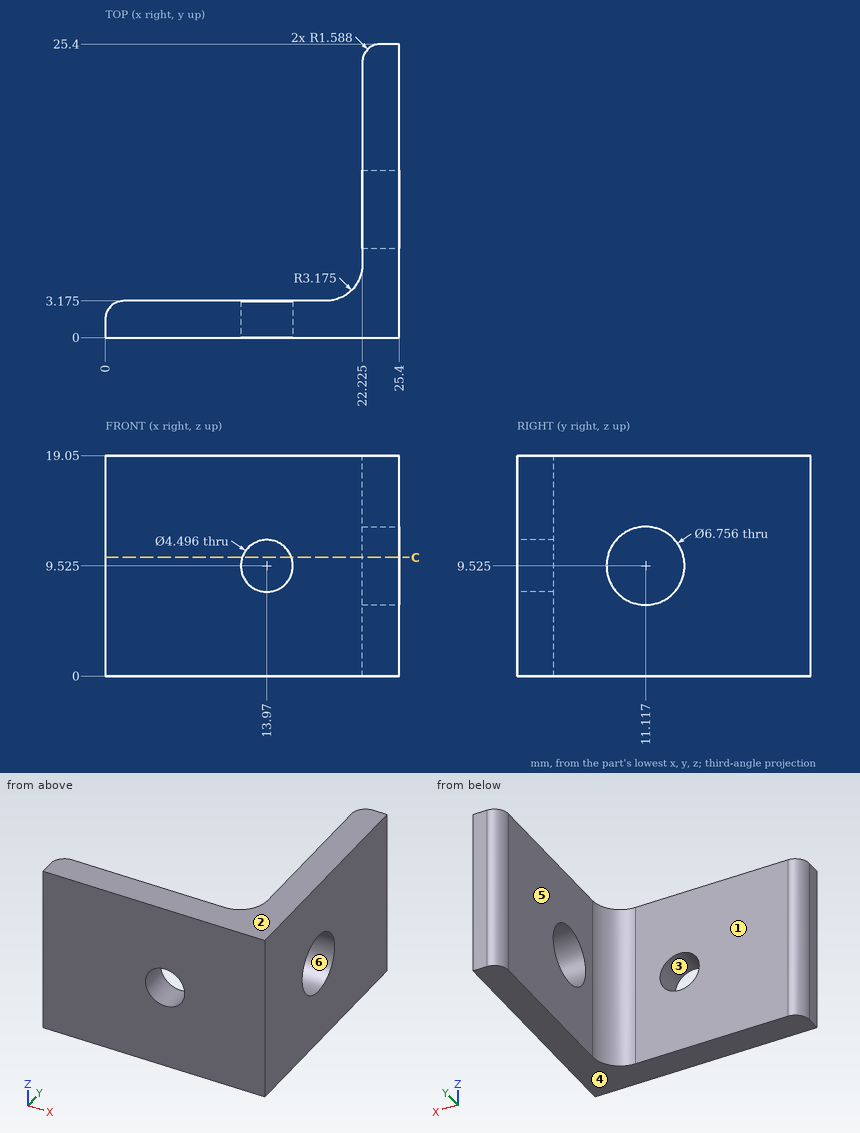
Part print with two shaded views. Sizes in mm from the minimum x, y, z corner. A direction names the side the tool comes from. Round coordinates to 2 decimals unless told otherwise and drop trailing zeros. Write each question's results on one line, items separated by ' | '.
1. Pull direction Z, two halves, no side cores. Call the marked faces 1, 2, 3 and 4: pulls with the +Z half, pulls with the -Z half, needs draft (parallel to the pull), parting line crosses it, or undercut.
Findings below:
face 1: needs draft | face 2: pulls with the +Z half | face 3: undercut | face 4: pulls with the -Z half
2. Wall check: line 1 along Z through (x, y) = (13.97, 1.1); line 2 along Y through (x, z) = (9.5, 14.5) (1 decimal); line 3 along X through (y, z) = (23, 3.75) (1 decimal). Give the ranges that are in metal, low to high. Write a range as [from, to].
Findings below:
line 1: z = [0, 7.28], [11.77, 19.05] | line 2: y = [0, 3.2] | line 3: x = [22.2, 25.4]
3. 3-axis set-ups, long thin cutter, end or side, ignore diameter. For the marked faces 5 and 6: which of +Z, -Z, +X, -X, +Y, -Y reach the whole face in a straight line?
Findings below:
face 5: +Z, -Z, -X, +Y | face 6: +X, -X
4. Flat gauge pins, fed straight in: P1, Ø2, axis at x = 22.5, z = 9, coming from the +Y side; P2, Ø8.5, axis at y = 12, z = 10, coming from the -X side (1 decimal); P3, Ø3, axis at x = 5.5, z = 2, coming from the +Y side (1 decimal). Where does each tip first touch, or does it go through?
Findings below:
P1: stops at y = 25.37 | P2: stops at x = 22.2 | P3: stops at y = 3.2
5. Cut at C-C (z = 10.25). Count the separate pieces of the cut face and the enclosed holes in it, plus the area to 3 significant figures.
Findings below:
separate pieces: 3 | enclosed holes: 0 | area: 118 mm²
